Check sheet for the modelled part. Datum: model origin and axes. Units: mm. A direction names the side the tool comes from. Round coordinates to 2 decimals unless told otherwise and drop trailing zeros. Order: outer loops, then holes, each group sorted by start corner. A loop starts at its lowest first (then second) coordinate and runs counter-clockwise, first axis right, second up. Notation, with made-up numbers: M 52.5,30.25 L 58.5,30.25 A34 ccw 58.5,63.25 Z; hole C 47.5,-23 d4. An arc over 180 degrees is marked long. One line per item, written item: value. Start each with the question number.
(1) Cross-section at C-C, the plane x = -104.5. Enter the section's corners in (y, z), and give its area (3 significant figures).
(2) Cross-section at D-D, the plane z = -40.5. Enter the section's corners in (x, y).
(3) Cross-section at B-B, the plane y = 115. Enter the section's corners in (x, z).
(4) Cross-section at A-A, the plane x = -147.75. Enter the section's corners in (y, z).
(5) Release check for a two-part mould opening along Y. For faces 3 (the face through (-110, 110, -41)), 4 (the face through (-71.2, 115.23, -90.14)), 5 (the face through (-109, 128, -80)) record: released by +Y, released by -Y, zero draft, split by the parting line, or undercut.
(6) Access from +Z, -Z, +X, -X, +Y, -Y to the whole of each face (thin tool, end or side, straight path). Record for faces 1 (the face through (-59.5, 105, -62)), 2 (the face through (-145, 110, -95)).
(7) Thickness scan on L1, parallel to X at y = 126.75, z = -85.75; L2, parallel to X at y = 115, z = -91; L3, parallel to Y at x = -147.75, z = -86. Record the ranges inside material, lowest first.
(8) Depth check by flat-ended pin: pin 1 Ø8 at (x, z) = (-71, -40) entering from +Y; pin 2 Ø4 at (x, y) = (-104.5, 135) entering from +Z; pin 3 Ø9 at (x, y) = (-143, 128) entering from -Z. Enter the tip coordinate at first touch or a pass-through.
Autodesk Inventor part; units mm, degrees
ref_plane "YZ Plane" through (0, 0, 0) normal (1, 0, 0) x (0, 1, 0)
ref_plane "XZ Plane" through (0, 0, 0) normal (0, 1, 0) x (-1, 0, 0)
ref_plane "XY Plane" through (0, 0, 0) normal (0, 0, 1) x (1, 0, 0)
sketch "Boceto2" plane through (0, 0, 0) normal (0, 1, 0) x (-1, 0, 0)
  line L0 (7.5, 100) -> (-7.5, 100)
  line L1 (-7.5, 100) -> (-7.5, -100)
  line L2 (-7.5, -100) -> (7.5, -100)
  line L3 (7.5, -100) -> (7.5, 100)
  line L4 (7.5, 100) -> (-7.5, -100) construction
  line L5 (-7.5, 100) -> (7.5, -100) construction
  point P0 (0, 0)
  dimension "d7" = 15
  dimension "d8" = 200
extrude "Extrusión1" add sketch "Boceto2" along normal blind 10
sketch "Boceto3" plane through (0, 10, 0) normal (0, 1, 0) x (1, 0, 0)
  line L0 (5, 60) -> (-5, 60)
  line L1 (-5, 60) -> (-5, 70)
  line L2 (-5, 70) -> (5, 70)
  line L3 (5, 70) -> (5, 60)
  line L4 (5, 60) -> (-5, 70) construction
  line L5 (7.5, 100) -> (-7.5, 100)
  line L6 (0, 64.5148) -> (0, 61.9205)
  circle A0 centre (3.25, 61.75) radius 1.75
  circle A1 centre (-3.25, 68.25) radius 1.75
  line L7 (-7.5, 100) -> (-7.5, -100)
  line L8 (-7.5, 0) -> (0, 0)
  line L9 (5, -70) -> (5, -60)
  line L10 (-5, -70) -> (5, -70)
  line L11 (5, -60) -> (-5, -60)
  line L12 (-5, -60) -> (-5, -70)
  line L13 (5, -60) -> (-5, -70) construction
  line L14 (0, -64.5148) -> (0, -61.9205)
  circle A2 centre (-3.25, -68.25) radius 1.75
  circle A3 centre (3.25, -61.75) radius 1.75
  point P0 (3.25, 68.25)
  point P1 (-5, 65)
  point P2 (-3.25, 61.75)
  point P3 (0, 100)
  point P4 (3.25, -68.25)
  point P5 (-3.25, -61.75)
  point P6 (-5, -65)
  dimension "d12" = 1.75
  dimension "d13" = 1.75
  dimension "d14" = 1.75
  dimension "d15" = 1.75
  dimension "d16" = 10
  dimension "d17" = 10
  dimension "d19" = 30
  dimension "d67" = 31.75
hole "Agujero1" at (3.25, 10, -61.75) at (-3.25, 10, -68.25) at (-3.25, 10, 68.25) at (3.25, 10, 61.75) direction (0, -1, 0) diameter 3.5 end through all
sketch "Boceto4" plane through (0, 10, 0) normal (0, 1, 0) x (1, 0, 0)
  line L0 (-7.5, 100) -> (-7.5, -100)
  line L1 (-7.5, -100) -> (7.5, -100)
  line L2 (7.5, -100) -> (7.5, -80)
  line L3 (7.5, -80) -> (-7.5, -80)
  line L4 (-7.5, -80) -> (-7.5, -100)
  line L5 (-7.5, 0) -> (1.0116, 0)
  line L6 (-7.5, -100) -> (-7.5, 100)
  line L7 (-7.5, 100) -> (7.5, 100)
  line L8 (7.5, 100) -> (7.5, 80)
  line L9 (7.5, 80) -> (-7.5, 80)
  line L10 (-7.5, 80) -> (-7.5, 100)
  point P0 (0, 0)
  point P1 (-7.5, -80)
  point P2 (-7.5, 80)
  dimension "d27" = 15
  dimension "d28" = 20
extrude "Extrusión2" add sketch "Boceto4" along normal blind 80
sketch "Boceto5" plane through (0, 90, 0) normal (0, 1, 0) x (1, 0, 0)
  line L0 (-7.5, -100) -> (7.5, -100)
  line L1 (-7.5, -100) -> (40.5, -100)
  line L2 (40.5, -100) -> (40.5, 100)
  line L3 (40.5, 100) -> (-7.5, 100)
  line L4 (-7.5, 100) -> (-7.5, -100)
  line L5 (40.5, -100) -> (-159.5, -100)
  line L6 (-159.5, -100) -> (-159.5, 100)
  line L7 (-159.5, 100) -> (40.5, 100)
  line L8 (40.5, 100) -> (40.5, -100)
  point P0 (0, 0)
  point P1 (-7.5, 100)
  dimension "d31" = 48
  dimension "d32" = 200
  dimension "d74" = 200
extrude "Extrusión3" add sketch "Boceto5" along normal blind 110
sketch "Boceto6" plane through (0, 200, 0) normal (0, 1, 0) x (1, 0, 0)
  line L0 (40.5, 100) -> (7.5, 100)
  line L1 (40.5, 100) -> (20.5, 100)
  line L2 (20.5, 100) -> (20.5, 80)
  line L3 (7.5, -100) -> (40.5, -100)
  line L4 (24, -100) -> (24, -80)
  line L5 (-159.5, 100) -> (-159.5, -100)
  line L6 (20.5, 80) -> (-159.5, 80)
  line L7 (-159.5, 80) -> (-159.5, -80)
  line L8 (-159.5, -80) -> (20.5, -80)
  line L9 (20.5, -80) -> (20.5, 80)
  line L10 (-159.5, -100) -> (40.5, -100)
  point P0 (7.5, 80)
  point P1 (-159.5, 80)
  dimension "d36" = 20
  dimension "d37" = 20
  dimension "d38" = 20
  dimension "d78" = 20
extrude "Extrusión4" cut sketch "Boceto6" against normal blind 90
sketch "Boceto7" plane through (-159.5, 90, -100) normal (-1, 0, 0) x (0, 0, 1)
  line L0 (0, 110) -> (20, 110)
  line L1 (20, 110) -> (10, 110)
  line L2 (10, 110) -> (10, 20)
  line L3 (10, 20) -> (20, 20)
  line L4 (20, 20) -> (20, 110)
  line L5 (180, 110) -> (180, 20)
  line L6 (180, 110) -> (190, 110)
  line L7 (190, 110) -> (190, 20)
  line L8 (190, 20) -> (180, 20)
  line L9 (180, 20) -> (180, 110)
  line L10 (200, 0) -> (200, 110)
  line L11 (0, 0) -> (0, 110)
  line L12 (0, 110) -> (10, 110)
  line L13 (10, 110) -> (10, 20)
  line L14 (10, 20) -> (0, 20)
  line L15 (0, 20) -> (0, 110)
  line L16 (200, 110) -> (0, 110)
  line L17 (200, 110) -> (190, 110)
  line L18 (190, 110) -> (190, 20)
  line L19 (190, 20) -> (200, 20)
  line L20 (200, 20) -> (200, 110)
  point P0 (100, -90)
  point P1 (200, 20)
  dimension "d42" = 10
  dimension "d63" = 10
  dimension "d65" = 10
extrude "Extrusión5" cut sketch "Boceto7" against normal blind 30 contours L0 L2 L14 L11 | L16 L10 L19 L7
sketch "Boceto8" plane through (-7.5, 0, 100) normal (0, 0, 1) x (1, 0, 0)
  line L0 (-122, 200) -> (-122, 110)
  line L1 (-132, 175) -> (-142, 175)
  line L2 (-142, 175) -> (-142, 185)
  line L3 (-142, 185) -> (-132, 185)
  line L4 (-132, 185) -> (-132, 175)
  line L5 (-132, 175) -> (-142, 185) construction
  line L6 (-142, 175) -> (-132, 185) construction
  line L7 (-152, 200) -> (48, 200)
  line L8 (-113, 155) -> (-128, 155)
  line L9 (-152, 110) -> (-122, 110)
  line L10 (-132, 180) -> (-131.5898, 180)
  circle A0 centre (-140.25, 183.25) radius 1.75
  circle A1 centre (-133.75, 176.75) radius 1.75
  line L11 (-132, 125) -> (-132, 135)
  line L12 (-142, 125) -> (-132, 125)
  line L13 (-132, 135) -> (-142, 125) construction
  line L14 (-132, 135) -> (-142, 135)
  line L15 (-142, 135) -> (-132, 125) construction
  line L16 (-142, 135) -> (-142, 125)
  line L17 (-132, 130) -> (-131.5898, 130)
  circle A2 centre (-133.75, 133.25) radius 1.75
  circle A3 centre (-140.25, 126.75) radius 1.75
  line L18 (-152, 110) -> (-152, 200)
  point P0 (7.5, 0)
  point P1 (-113, 215)
  point P2 (-133.75, 183.25)
  point P3 (-142, 180)
  point P4 (-140.25, 176.75)
  point P5 (48, 200)
  point P6 (-133.75, 126.75)
  point P7 (-140.25, 133.25)
  point P8 (-143, 115)
  point P9 (-133.75, 126.75)
  point P10 (-140.25, 133.25)
  point P11 (-142, 130)
  dimension "d46" = 1.75
  dimension "d47" = 1.75
  dimension "d48" = 1.75
  dimension "d49" = 1.75
  dimension "d50" = 10
  dimension "d51" = 10
  dimension "d52" = 15
  dimension "d66" = 10
  dimension "d70" = 15
hole "Agujero2" at (-147.75, 183.25, 100) at (-141.25, 176.75, 100) at (-147.75, 126.75, 100) at (-141.25, 133.25, 100) direction (0, 0, -1) diameter 3.5 end through all
ref_plane "Plano de trabajo1" through (-159.5, 90, 100) normal (0, -1, 0) x (1, 0, 0)
split "Dividir1" plane through (-159.5, 90, 100) removes the side toward (0, -1, 0)
ref_plane "Plano de trabajo2" through (-159.5, 200, 0) normal (0, 0, 1) x (1, 0, 0)
ref_plane "Plano de trabajo3" through (-59.5, 90, 100) normal (1, 0, 0) x (0, 0, -1)
sketch "Boceto9" plane through (-159.5, 90, 100) normal (0, 0, 1) x (1, 0, 0)
  line L0 (85.0357, 30) -> (115.0357, 30)
  circle A0 centre (110.0357, 25) radius 1.75
  line L1 (90.0357, 25) -> (110.0357, 25)
  line L2 (115.0357, 30) -> (115.0357, 20)
  circle A1 centre (90.0357, 25) radius 1.75
  line L3 (85.0357, 20) -> (115.0357, 30) construction
  line L4 (85.0357, 30) -> (115.0357, 20) construction
  line L5 (85.0357, 20) -> (85.0357, 30)
  line L6 (115.0357, 20) -> (85.0357, 20)
  line L7 (240, 0) -> (-40, 0)
  line L8 (200, 0) -> (200, 110)
  line L9 (200, 55) -> (88.2857, 55)
  line L10 (85.0357, 80) -> (115.0357, 80)
  circle A2 centre (110.0357, 85) radius 1.75
  line L11 (90.0357, 85) -> (110.0357, 85)
  line L12 (115.0357, 80) -> (115.0357, 90)
  circle A3 centre (90.0357, 85) radius 1.75
  line L13 (85.0357, 90) -> (115.0357, 80) construction
  line L14 (85.0357, 80) -> (115.0357, 90) construction
  line L15 (85.0357, 90) -> (85.0357, 80)
  line L16 (115.0357, 90) -> (85.0357, 90)
  line L17 (100.0357, 55) -> (185.099, 55) construction
  line L18 (160, 70) -> (160, 40)
  circle A4 centre (165, 45) radius 1.75
  line L19 (165, 65) -> (165, 45)
  line L20 (160, 40) -> (170, 40)
  circle A5 centre (165, 65) radius 1.75
  line L21 (170, 70) -> (160, 40) construction
  line L22 (160, 70) -> (170, 40) construction
  line L23 (170, 70) -> (160, 70)
  line L24 (170, 40) -> (170, 70)
  circle A6 centre (55, 65) radius 1.75
  line L25 (60, 70) -> (60, 40)
  line L26 (60, 70) -> (50, 40) construction
  line L27 (50, 70) -> (60, 70)
  line L28 (50, 40) -> (50, 70)
  line L29 (50, 70) -> (60, 40) construction
  circle A7 centre (55, 45) radius 1.75
  line L30 (55, 65) -> (55, 45)
  line L31 (60, 40) -> (50, 40)
  line L32 (30, 110) -> (30, 20)
  point P0 (159.5, -90)
  point P1 (100.0357, 34.7141)
  point P2 (85.0357, 36.6749)
  point P3 (100.0357, 34.7141)
  point P4 (115.0357, 25)
  point P5 (115.0357, 85)
  point P6 (189.1833, 40)
  point P7 (165, 70)
  point P8 (70.0357, 40)
  point P9 (55, 70)
  dimension "d83" = 10
  dimension "d84" = 30
  dimension "d85" = 5
  dimension "d86" = 5
  dimension "d87" = 5
  dimension "d88" = 5
  dimension "d89" = 20
  dimension "d91" = 30
  dimension "d92" = 5
  dimension "d93" = 5
  dimension "d94" = 3.5
  dimension "d95" = 5
  dimension "d96" = 5
  dimension "d97" = 5
  dimension "d98" = 5
  dimension "d99" = 5
  dimension "d100" = 20
ref_plane "Plano de trabajo4" through (0, 145, 0) normal (0, 1, 0) x (1, 0, 0)
hole "Agujero3" at (-104.5, 155, 100) at (-69.4643, 175, 100) at (-49.4643, 175, 100) at (-104.5, 135, 100) at (-69.4643, 115, 100) at (-49.4643, 115, 100) at (5.5, 135, 100) at (5.5, 155, 100) direction (0, 0, -1) diameter 3.5 end through all
sketch "Boceto10" plane through (40.5, 90, 100) normal (1, 0, 0) x (0, 0, -1)
  line L0 (85.0357, 30) -> (115.0357, 30)
  circle A0 centre (110.0357, 25) radius 1.75
  line L1 (90.0357, 25) -> (110.0357, 25)
  line L2 (115.0357, 30) -> (115.0357, 20)
  circle A1 centre (90.0357, 25) radius 1.75
  line L3 (85.0357, 20) -> (115.0357, 30) construction
  line L4 (85.0357, 30) -> (115.0357, 20) construction
  line L5 (85.0357, 20) -> (85.0357, 30)
  line L6 (115.0357, 20) -> (85.0357, 20)
  circle A2 centre (90.0357, 85) radius 1.75
  line L7 (85.0357, 80) -> (115.0357, 80)
  line L8 (85.0357, 80) -> (115.0357, 90) construction
  line L9 (85.0357, 90) -> (85.0357, 80)
  line L10 (115.0357, 90) -> (85.0357, 90)
  line L11 (85.0357, 90) -> (115.0357, 80) construction
  circle A3 centre (110.0357, 85) radius 1.75
  line L12 (90.0357, 85) -> (110.0357, 85)
  line L13 (115.0357, 80) -> (115.0357, 90)
  line L14 (160, 70) -> (160, 40)
  circle A4 centre (165, 45) radius 1.75
  line L15 (170, 40) -> (170, 70)
  line L16 (170, 70) -> (160, 40) construction
  line L17 (160, 40) -> (170, 40)
  line L18 (160, 70) -> (170, 40) construction
  circle A5 centre (165, 65) radius 1.75
  line L19 (165, 65) -> (165, 45)
  line L20 (170, 70) -> (160, 70)
  circle A6 centre (35, 65) radius 1.75
  line L21 (40, 70) -> (40, 40)
  line L22 (40, 40) -> (30, 40)
  circle A7 centre (35, 45) radius 1.75
  line L23 (35, 65) -> (35, 45)
  line L24 (40, 70) -> (30, 40) construction
  line L25 (30, 40) -> (30, 70)
  line L26 (30, 70) -> (40, 40) construction
  line L27 (30, 70) -> (40, 70)
  line L28 (0, 0) -> (0, 110)
  line L29 (200, 0) -> (200, 110)
  point P0 (100, -90)
  point P1 (100.0357, 34.7141)
  point P2 (100.0357, 34.7141)
  point P3 (85.0357, 36.6749)
  point P4 (115.0357, 25)
  point P5 (88.2857, 55)
  point P6 (115.0357, 85)
  point P7 (100.0357, 55)
  point P8 (189.1833, 40)
  point P9 (165, 70)
  point P10 (70.0357, 40)
  point P11 (35, 70)
  dimension "d108" = 10
  dimension "d109" = 30
  dimension "d110" = 5
  dimension "d111" = 5
  dimension "d112" = 5
  dimension "d113" = 5
  dimension "d114" = 5
  dimension "d115" = 5
  dimension "d116" = 3.5
  dimension "d117" = 5
  dimension "d118" = 5
  dimension "d119" = 5
  dimension "d120" = 5
  dimension "d121" = 5
  dimension "d122" = 30
  dimension "d123" = 30
hole "Agujero4" at (40.5, 175, 9.9643) at (40.5, 175, -10.0357) at (40.5, 155, 65) at (40.5, 135, 65) at (40.5, 115, 9.9643) at (40.5, 115, -10.0357) at (40.5, 135, -65) at (40.5, 155, -65) direction (-1, 0, 0) diameter 3.5 end through all
split "Dividir2" plane through (-59.5, 90, 100) removes the side toward (1, 0, 0)
split "Dividir3" plane through (0, 145, 0) removes the side toward (0, 1, 0)
split "Dividir4" plane through (-159.5, 200, 0) removes the side toward (0, 0, 1)
properties part number "container_back_head_3"
Values found:
1. outline: M 90,-100 L 133.25,-100 L 133.25,-80 L 110,-80 L 110,0 L 90,0 Z; M 136.75,-100 L 145,-100 L 145,-80 L 136.75,-80 Z
1. area: 2,630 mm^2
2. outline: M -159.5,90 L -59.5,90 L -59.5,110 L -159.5,110 Z
3. outline: M -159.5,-90 L -129.5,-90 L -129.5,-100 L -71.21,-100 L -71.21,-80 L -159.5,-80 Z; M -67.71,-100 L -59.5,-100 L -59.5,-80 L -67.71,-80 Z
4. outline: M 90,-100 L 110,-100 L 110,-90 L 125,-90 L 125,-80 L 110,-80 L 110,0 L 90,0 Z; M 128.5,-90 L 145,-90 L 145,-80 L 128.5,-80 Z
5. face 3: released by +Y
5. face 4: undercut
5. face 5: zero draft
6. face 1: +Z, -Z, +X, +Y, -Y
6. face 2: -Z, -X, +Y
7. L1: -159.5 to -149.5, -146 to -59.5
7. L2: -129.5 to -71.21, -67.71 to -59.5
7. L3: 90 to 125, 128.5 to 145
8. pin 1: y = 110
8. pin 2: z = -80
8. pin 3: z = -90
